from build123d import *

# Parameters (mm, degrees)
BOSS_EXTRUDE1_DEPTH = 3
SKETCH4_R           = 0.2
CUT_EXTRUDE1_DEPTH  = 13.5


with BuildPart() as part:
    # Sketch2 → Revolve1 (revolve)
    with BuildSketch(Plane.XY):
        Polygon((3, 12.5), (0, 12.5), (0, 0), (0.5, 0), (1.900415076, 2), (3.5, 2), (3.5, 5), (2.5, 5), (2.5, 6.5), (3, 6.5), align=None)
    revolve(axis=Axis((0, 12.5, 0), (0, -1, 0)))

    # Sketch3 → Boss-Extrude1 (add)
    with BuildSketch(Plane.XZ.offset(-2)):
        Polygon((-4.020157505, 0.41432713), (-2.368896572, -3.274394961), (1.651260932, -3.688722091), (4.020157505, -0.41432713), (2.368896572, 3.274394961), (-1.651260932, 3.688722091), align=None)
    extrude(amount=-BOSS_EXTRUDE1_DEPTH)

    # Sketch4 → Cut-Extrude1 (cut, through all)
    with BuildSketch(Plane.XZ):
        Circle(SKETCH4_R)
    extrude(amount=-CUT_EXTRUDE1_DEPTH, mode=Mode.SUBTRACT)


solid = part.part
Can you work these out from the model? Positions are in its coordinate system, mm. A direction names the side the tool comes from. Give positions to 0.01 mm unless a question says otherwise; leave off trailing zeros. Loops run counter-clockwise (first coordinate to the right, second up) from the corner with the lowest first, then second, coordinate; pieces in that order, holes last. Notation, with made-up numbers: M 56,59.5 L 95,59.5 A11 cw 95,75.5 Z; hole C 88.5,80.5 d2. An arc over 180 degrees is marked long. One line per item, written item: value. Start each with the question number.
1) If we section it at D-D, the plane z = 2.25: Write out the boundary of the cut face in (x, y).
2) On a 3-axis mill with a long thin cutter (end or side, diameter ignored), from which of +Z, -Z, +X, -X, +Y, -Y can I reach the whole of each face in a straight line? I mean faces 1 (the face through (-1, 2, 2)), 2 (the face through (-3, 10, 0)), 3 (the face through (-0.39, 3.48, -3.48)), 4 (the face through (2, 6.5, 2)), 5 (the face through (-2.8, 3.5, 2.1)). Say none if no direction works.
3) If we section it at A-A, the plane y = 3.25: Write out the boundary of the cut face in (x, z), and give its area (3 significant figures).
4) If I drill on line 1 (Z direction, x = 0, y = 9.5); line 2 (Z direction, x = 0, y = 5.5); line 3 (Z direction, x = -2.75, y = 3.75), over which ranges is the centre line in solid material (lowest first)? Write a range as [from, to].
5) I'm going to push flat-ended pins straight in: pin 1 (2 mm diameter, centred on x = -1, z = -1.5, fed in from -Y); pin 2 (4 mm diameter, centred on x = 3, y = 9, fed in from -Z); pin 3 (2 mm diameter, centred on x = -0.5, y = 1.5, fed in from -Z). Where does each tip first touch, or does it pass through?
6) If we section it at C-C, the plane z = 0: Write out the boundary of the cut face in (x, y), and give its area (3 significant figures).
7) If we section it at B-B, the plane x = 0: Write out the boundary of the cut face in (y, z).
8) Thinking about a two-plate mould opening in Y: for faces 6 (the face through (1, 12.5, 0)), 7 (the face through (-0.54, 5.76, -2.44)), 8 (the face through (-3.21, 3.48, -1.4)), which applies, +Y half, -Y half, draft (parallel to the pull), parting line (faces both ways), or undercut?
Completed:
1. outline: M -2.69,2 L 2.83,2 L 2.83,5 L 1.09,5 L 1.09,6.5 L 1.98,6.5 L 1.98,12.5 L -1.98,12.5 L -1.98,6.5 L -1.09,6.5 L -1.09,5 L -2.69,5 Z
2. face 1: -Y
2. face 2: +Y
2. face 3: -Z, -X, +Y, -Y
2. face 4: none
2. face 5: +Z, -X, +Y, -Y
3. outline: M -4.02,0.41 L -2.37,-3.27 L 1.65,-3.69 L 4.02,-0.41 L 2.37,3.27 L -1.65,3.69 Z; hole C 0,0 d0.4
3. area: 42.3 mm^2
4. line 1: z = [-3, -0.2], [0.2, 3]
4. line 2: z = [-2.5, -0.2], [0.2, 2.5]
4. line 3: z = [-2.42, 2.17]
5. pin 1: stops at y = 0.43
5. pin 2: stops at z = -2.83
5. pin 3: stops at z = -3.56
6. outline: M -3.83,2 L -1.9,2 L -0.5,0 L -0.2,0 L -0.2,12.5 L -3,12.5 L -3,6.5 L -2.5,6.5 L -2.5,5 L -3.83,5 Z; M 0.2,0 L 0.5,0 L 1.9,2 L 3.83,2 L 3.83,5 L 2.5,5 L 2.5,6.5 L 3,6.5 L 3,12.5 L 0.2,12.5 Z
6. area: 66.3 mm^2
7. outline: M 0,-0.5 L 2,-1.9 L 2,-3.52 L 5,-3.52 L 5,-2.5 L 6.5,-2.5 L 6.5,-3 L 12.5,-3 L 12.5,-0.2 L 0,-0.2 Z; M 0,0.2 L 12.5,0.2 L 12.5,3 L 6.5,3 L 6.5,2.5 L 5,2.5 L 5,3.52 L 2,3.52 L 2,1.9 L 0,0.5 Z
8. face 6: +Y half
8. face 7: undercut
8. face 8: draft
